from build123d import *

# Parameters (mm, degrees)
F0_R          = 1.5875
F0_R_2        = 1.016
F1_DEPTH      = 15.875
F2_DEPTH      = 3.175
F2_DEPTH_BACK = 15.875
F3_SIZE       = 0.254


with BuildPart() as f1:
    # F0 (on Front) → F1 (new body)
    with BuildSketch(Plane.XZ):
        Circle(F0_R)
        Circle(F0_R_2, mode=Mode.SUBTRACT)
    extrude(amount=-F1_DEPTH)

    # F0 (on Front) → F2 (join, two sides)
    with BuildSketch(Plane.XZ) as f2_sk:
        Circle(F0_R_2)
    extrude(amount=F2_DEPTH)
    extrude(f2_sk.sketch, amount=-F2_DEPTH_BACK)

    # F3
    f3_edges = [f1.edges().sort_by_distance(p)[0] for p in [
        (-1.5875, 15.875, 0),
        (-1.016, -3.175, 0),
    ]]
    chamfer(f3_edges, length=F3_SIZE)


solid = f1.part
Here's how the part is built. I have some questions about the finished solid (model axes, mm). A direction names the side the tool comes from. Coordinates: 2 decimals unless noted, no trailing zeros. Order: outer loops, then holes, each group sorted by start corner. A loop starts at its lowest first (then second) coordinate and runs counter-clockwise, first axis right, second up.
Item 1: If we section it at C-C on y = 8: List the corners of the cut face in (x, z) for me (1 decimal).
Result sheet:
outline: circle Ø3.2 at (0, 0)
Item 2: For faces 1 (the face through (-0.22, -1.44, -0.99)), 2 (the face through (0, -3.175, 0)), which set-ups out of +Z, -Z, +X, -X, +Y, -Y let a thin tool reach every point of the face, with its end or its side?
Result sheet:
face 1: -Y
face 2: +Z, -Z, +X, -X, -Y
Item 3: I need wall thicknesses on line 1 (Z direction, x = 0.1, y = 3); line 2 (Z direction, x = 0.55, y = 12); line 3 (X direction, y = 14.25, z = 1.25). Which ranges of each line are inside material? Lowest first, please.
Result sheet:
line 1: z = -1.58 to 1.58
line 2: z = -1.49 to 1.49
line 3: x = -0.98 to 0.98
